```python
from build123d import *

# Parameters (mm, degrees)
F0_W     = 3.0607780209
F0_H     = 2.1009956449
F1_DEPTH = 5
F3_DEPTH = 2
F4_START = -3
F4_DEPTH = 2


with BuildPart() as f1:
    # F0 (on Front) → F1 (new body)
    with BuildSketch(Plane.XZ):
        with BuildLine():
            Line((-13.4510826319, 3.0807058793), (-20.9973859143, 3.0807058793))
            Line((-20.9973859143, 3.0807058793), (-26.770388545, -8.5309240967))
            Line((-26.770388545, -8.5309240967), (-26.3940021396, -8.5309240967))
            Line((-26.3940021396, -8.5309240967), (-26.3940021396, -9.6365026161))
            Line((-26.3940021396, -9.6365026161), (-21.3870331645, -9.6365026161))
            Line((-21.3870331645, -9.6365026161), (-21.3870331645, -11.8402632847))
            Line((-21.3870331645, -11.8402632847), (-24.6597826481, -11.8402632847))
            Line((-24.6597826481, -11.8402632847), (-24.6597826481, -10.3107876107))
            Line((-24.6597826481, -10.3107876107), (-26.3940021396, -10.3107876107))
            Line((-26.3940021396, -10.3107876107), (-26.3940021396, -12.9192377403))
            Line((-26.3940021396, -12.9192377403), (-20.359800871, -12.9192377403))
            ThreePointArc((-20.359800871, -12.9192377403), (-19.8294707851, -12.6995678262), (-19.609800871, -12.1692377403))
            Line((-19.609800871, -12.1692377403), (-19.609800871, -9.2809240967))
            ThreePointArc((-19.609800871, -9.2809240967), (-19.8294707851, -8.7505940108), (-20.359800871, -8.5309240967))
            Line((-20.359800871, -8.5309240967), (-19.2351932671, -8.5309240967))
            Line((-19.2351932671, -8.5309240967), (-16.9493351132, -3.8456239272))
            Line((-16.9493351132, -3.8456239272), (-13.144302211, -8.5309240967))
            Line((-13.144302211, -8.5309240967), (-14.130868949, -8.5309240967))
            Line((-14.130868949, -8.5309240967), (-14.130868949, -11.8141257167))
            Line((-14.130868949, -11.8141257167), (-17.3050090671, -11.8141257167))
            Line((-17.3050090671, -11.8141257167), (-17.3050090671, -8.5309240967))
            Line((-17.3050090671, -8.5309240967), (-19.167387858, -8.5309240967))
            Line((-19.167387858, -8.5309240967), (-19.167387858, -12.1691745073))
            ThreePointArc((-19.167387858, -12.1691745073), (-18.9477179439, -12.6995045932), (-18.417387858, -12.9191745073))
            Line((-18.417387858, -12.9191745073), (-12.2846849263, -12.9191745073))
            Line((-12.2846849263, -12.9191745073), (-12.2846849263, -8.5309240967))
            Line((-12.2846849263, -8.5309240967), (-11.065042235, -8.5309240967))
            ThreePointArc((-11.065042235, -8.5309240967), (-11.5953723208, -8.7505940108), (-11.815042235, -9.2809240967))
            Line((-11.815042235, -9.2809240967), (-11.815042235, -12.1692377403))
            ThreePointArc((-11.815042235, -12.1692377403), (-11.5953723208, -12.6995678262), (-11.065042235, -12.9192377403))
            Line((-11.065042235, -12.9192377403), (-5.1752589643, -12.9192377403))
            Line((-5.1752589643, -12.9192377403), (-5.1752589643, -11.9112924635))
            Line((-5.1752589643, -11.9112924635), (-10.0498311222, -11.9112924635))
            Line((-10.0498311222, -11.9112924635), (-10.0498311222, -9.8059958741))
            Line((-10.0498311222, -9.8059958741), (-5.1752589643, -9.8059958741))
            Line((-5.1752589643, -9.8059958741), (-5.1752589643, -8.5309240967))
            Line((-5.1752589643, -8.5309240967), (-4.6894219704, -8.5309240967))
            Line((-4.6894219704, -8.5309240967), (-4.6894219704, -12.9192377403))
            Line((-4.6894219704, -12.9192377403), (-2.891822136, -12.9192377403))
            Line((-2.891822136, -12.9192377403), (-2.891822136, -11.6197903603))
            Line((-2.891822136, -11.6197903603), (0.1689558849, -11.6197903603))
            Line((0.1689558849, -11.6197903603), (0.1689558849, -12.9192377403))
            Line((0.1689558849, -12.9192377403), (2.096112119, -12.9192377403))
            Line((2.096112119, -12.9192377403), (2.096112119, -8.5309240967))
            Line((2.096112119, -8.5309240967), (2.4571896065, -8.5309240967))
            Line((2.4571896065, -8.5309240967), (7.3034735397, -4.2975358665))
            Line((7.3034735397, -4.2975358665), (6.7291194573, -8.5309240967))
            Line((6.7291194573, -8.5309240967), (3.2661118247, -8.5309240967))
            ThreePointArc((3.2661118247, -8.5309240967), (2.7357817388, -8.7505940108), (2.5161118247, -9.2809240967))
            Line((2.5161118247, -9.2809240967), (2.5161118247, -12.1692377403))
            ThreePointArc((2.5161118247, -12.1692377403), (2.7357817388, -12.6995678262), (3.2661118247, -12.9192377403))
            Line((3.2661118247, -12.9192377403), (9.1558950953, -12.9192377403))
            Line((9.1558950953, -12.9192377403), (9.1558950953, -11.9984643534))
            Line((9.1558950953, -11.9984643534), (4.2813229375, -11.9984643534))
            Line((4.2813229375, -11.9984643534), (4.2813229375, -11.445844546))
            Line((4.2813229375, -11.445844546), (8.6850486696, -11.445844546))
            Line((8.6850486696, -11.445844546), (8.6850486696, -10.4135535657))
            Line((8.6850486696, -10.4135535657), (4.2813229375, -10.4135535657))
            Line((4.2813229375, -10.4135535657), (4.2813229375, -9.805932641))
            Line((4.2813229375, -9.805932641), (9.1558950953, -9.805932641))
            Line((9.1558950953, -9.805932641), (9.1558950953, -8.5309240967))
            Line((9.1558950953, -8.5309240967), (10.1831596047, -8.5309240967))
            ThreePointArc((10.1831596047, -8.5309240967), (9.6528295188, -8.7505940108), (9.4331596047, -9.2809240967))
            Line((9.4331596047, -9.2809240967), (9.4331596047, -10.550885953))
            ThreePointArc((9.4331596047, -10.550885953), (9.6528295188, -11.0812160389), (10.1831596047, -11.300885953))
            Line((10.1831596047, -11.300885953), (14.1622014344, -11.300885953))
            Line((14.1622014344, -11.300885953), (14.1622014344, -11.9984643534))
            Line((14.1622014344, -11.9984643534), (9.4331596047, -11.9984643534))
            Line((9.4331596047, -11.9984643534), (9.4331596047, -12.9191745073))
            Line((9.4331596047, -12.9191745073), (15.0284558833, -12.9191745073))
            ThreePointArc((15.0284558833, -12.9191745073), (15.5587859692, -12.6995045932), (15.7784558833, -12.1691745073))
            Line((15.7784558833, -12.1691745073), (15.7784558833, -11.1678693146))
            ThreePointArc((15.7784558833, -11.1678693146), (15.5587859692, -10.6375392287), (15.0284558833, -10.4178693146))
            Line((15.0284558833, -10.4178693146), (11.2140327692, -10.4178693146))
            Line((11.2140327692, -10.4178693146), (11.2140327692, -9.7743598744))
            Line((11.2140327692, -9.7743598744), (15.7784558833, -9.7743598744))
            Line((15.7784558833, -9.7743598744), (15.7784558833, -8.5309240967))
            Line((15.7784558833, -8.5309240967), (12.7156563103, -8.5309240967))
            Line((12.7156563103, -8.5309240967), (17.5534840673, -4.2975358665))
            Line((17.5534840673, -4.2975358665), (17.0895829797, -8.5309240967))
            Line((17.0895829797, -8.5309240967), (17.0398395211, -8.5309240967))
            ThreePointArc((17.0398395211, -8.5309240967), (16.5095094352, -8.7505940108), (16.2898395211, -9.2809240967))
            Line((16.2898395211, -9.2809240967), (16.2898395211, -10.550885953))
            ThreePointArc((16.2898395211, -10.550885953), (16.5095094352, -11.0812160389), (17.0398395211, -11.300885953))
            Line((17.0398395211, -11.300885953), (21.0188813508, -11.300885953))
            Line((21.0188813508, -11.300885953), (21.0188813508, -11.9984643534))
            Line((21.0188813508, -11.9984643534), (16.2898395211, -11.9984643534))
            Line((16.2898395211, -11.9984643534), (16.2898395211, -12.9191745073))
            Line((16.2898395211, -12.9191745073), (21.8851357996, -12.9191745073))
            ThreePointArc((21.8851357996, -12.9191745073), (22.4154658855, -12.6995045932), (22.6351357996, -12.1691745073))
            Line((22.6351357996, -12.1691745073), (22.6351357996, -11.1678693146))
            ThreePointArc((22.6351357996, -11.1678693146), (22.4154658855, -10.6375392287), (21.8851357996, -10.4178693146))
            Line((21.8851357996, -10.4178693146), (18.0707126856, -10.4178693146))
            Line((18.0707126856, -10.4178693146), (18.0707126856, -9.7743598744))
            Line((18.0707126856, -9.7743598744), (22.6351357996, -9.7743598744))
            Line((22.6351357996, -9.7743598744), (22.6351357996, -8.5309240967))
            Line((22.6351357996, -8.5309240967), (23.4516598284, -8.5309240967))
            Line((23.4516598284, -8.5309240967), (25.7711652666, 3.0807058793))
            Line((25.7711652666, 3.0807058793), (19.431181252, 3.0807058793))
            Line((19.431181252, 3.0807058793), (14.2619935796, -1.4036741341))
            Line((14.2619935796, -1.4036741341), (15.0130717084, 3.0807058793))
            Line((15.0130717084, 3.0807058793), (9.1148968786, 3.0807058793))
            Line((9.1148968786, 3.0807058793), (1.9796516281, -3.5022755619))
            Line((1.9796516281, -3.5022755619), (5.0060558133, 4.4282288291))
            Line((5.0060558133, 4.4282288291), (15.0130717084, 4.4282288291))
            Line((15.0130717084, 4.4282288291), (15.7288057171, 6.8140071817))
            Line((15.7288057171, 6.8140071817), (-11.583940126, 6.8140071817))
            Line((-11.583940126, 6.8140071817), (-12.7105582505, 4.4282288291))
            Line((-12.7105582505, 4.4282288291), (-2.5268180761, 4.4282288291))
            Line((-2.5268180761, 4.4282288291), (-6.9228359498, -5.4683336057))
            Line((-6.9228359498, -5.4683336057), (-10.288979272, -1.3234569953))
            Line((-10.288979272, -1.3234569953), (-4.2719710618, 3.0807058793))
            Line((-4.2719710618, 3.0807058793), (-9.4190677628, 3.0807058793))
            Line((-9.4190677628, 3.0807058793), (-15.5823286623, -1.0281349532))
            Line((-15.5823286623, -1.0281349532), (-13.4510826319, 3.0807058793))
        make_face()
        with Locations((-1.3614331256, -9.5814219192)):
            Rectangle(F0_W, F0_H, mode=Mode.SUBTRACT)
    extrude(amount=F1_DEPTH)

    # F2 (on face) → F3 (cut)
    with BuildSketch(Plane.XZ.offset(5)):
        Polygon((-26.770388545, 6.8140071817), (-26.770388545, -8.5309240967), (26.5221912414, -8.5309240967), (26.5221912414, 6.8140071817), (13.7877286713, 6.8140071817), (7.3034735397, 6.8140071817), (5.1193437539, 6.8140071817), (4.2332103827, 6.8140071817), (2.1055981025, 6.8140071817), (-2.0268179942, 6.8140071817), (-4.4263883249, 6.8140071817), (-10.9106434565, 6.8140071817), align=None)
        Polygon((-5.7986674306, 17.639362709), (-10.9106434565, 6.8140071817), (-4.4263883249, 6.8140071817), (-1.1687912286, 13.7124446064), (-5.4921403697, 13.7124446064), (-4.4917744037, 15.8308655821), (-0.1684252625, 15.8308655821), (0.685587701, 17.639362709), align=None)
        Polygon((-7.9570718311, 8.492592384), (-6.3421407991, 11.9124446064), (-3.5912522867, 11.9124446064), (-5.2061833186, 8.492592384), align=None, mode=Mode.SUBTRACT)
        Polygon((7.3034735397, 6.8140071817), (13.7877286713, 6.8140071817), (18.8997046972, 17.639362709), (12.4154495655, 17.639362709), align=None)
        Polygon((10.0692709763, 8.492592384), (13.3818611683, 15.5074857175), (15.9919188063, 15.5074857175), (12.6793286143, 8.492592384), align=None, mode=Mode.SUBTRACT)
        Polygon((-0.6024195059, 9.8303789273), (-2.0268179942, 6.8140071817), (2.1055981025, 6.8140071817), (4.2332103827, 6.8140071817), (5.1193437539, 6.8140071817), (10.2313197798, 17.639362709), (3.0851580317, 17.639362709), (0.3012099711, 11.7439462647), (5.3197594389, 11.7439462647), (3.7843971086, 8.492592384), (0.9204373378, 8.492592384), (1.5521701913, 9.8303789273), align=None)
        Polygon((2.98915204, 13.6170848409), (3.9799346353, 15.7152116299), (7.1950801421, 15.7152116299), (6.2042975468, 13.6170848409), align=None, mode=Mode.SUBTRACT)
    extrude(amount=-F3_DEPTH, mode=Mode.SUBTRACT)

    # F2 (on face) → F4 (join)
    with BuildSketch(Plane.XZ.offset(5).offset(F4_START)):
        Polygon((-5.7986674306, 17.639362709), (-10.9106434565, 6.8140071817), (-4.4263883249, 6.8140071817), (-1.1687912286, 13.7124446064), (-5.4921403697, 13.7124446064), (-4.4917744037, 15.8308655821), (-0.1684252625, 15.8308655821), (0.685587701, 17.639362709), align=None)
        Polygon((-7.9570718311, 8.492592384), (-6.3421407991, 11.9124446064), (-3.5912522867, 11.9124446064), (-5.2061833186, 8.492592384), align=None, mode=Mode.SUBTRACT)
        Polygon((-0.6024195059, 9.8303789273), (-2.0268179942, 6.8140071817), (2.1055981025, 6.8140071817), (4.2332103827, 6.8140071817), (5.1193437539, 6.8140071817), (10.2313197798, 17.639362709), (3.0851580317, 17.639362709), (0.3012099711, 11.7439462647), (5.3197594389, 11.7439462647), (3.7843971086, 8.492592384), (0.9204373378, 8.492592384), (1.5521701913, 9.8303789273), align=None)
        Polygon((2.98915204, 13.6170848409), (3.9799346353, 15.7152116299), (7.1950801421, 15.7152116299), (6.2042975468, 13.6170848409), align=None, mode=Mode.SUBTRACT)
        Polygon((12.4154495655, 17.639362709), (7.3034735397, 6.8140071817), (13.7877286713, 6.8140071817), (18.8997046972, 17.639362709), align=None)
        Polygon((10.0692709763, 8.492592384), (13.3818611683, 15.5074857175), (15.9919188063, 15.5074857175), (12.6793286143, 8.492592384), align=None, mode=Mode.SUBTRACT)
    extrude(amount=-F4_DEPTH)


solid = f1.part
```
Design review of the part built by this model. Coordinates are the model's own, in mm. A direction names the side the tool comes from. Give positions to 0.01 mm unless a question says otherwise; leave off trailing zeros. Write each loop counter-clockwise with the first axis right and the second up, starting at its lowest first coordinate (ties: lowest second). Pieces come first, ordered by that corner, then holes. Notation, with made-up numbers: (-10, 48.5) - (44, 48.5) arc R19 ccw to (44, 52.5) - close; hole circle Ø9 at (-40, -36.5). An arc over 180 degrees is marked (long way). Return JSON: item names as keys, results as strings. Group by question number.
(1) Insertion check: pin 1 (5 mm diameter, centred on x = 16, z = 3.5, fed in from -Y); pin 2 (0.6 mm diameter, centred on y = -2.5, z = -12.5, fed in from +X); pin 3 (3 mm diameter, centred on y = -3, z = 3.5, fed in from -X). Each pin has a flat end and moves straight along its axis. Give the tip position at first contact, or say it passes through.
(2) To check wall thickness, follow probe 1 along Z at (x, y) = (20, -0.35); probe 2 along Z at (x, y) = (11, -4.4); probe 3 along X at (y, z) = (-0.45, 14.5). State the ranges of each line that lie inside material, in increasing order.
(3) We need section A-A, the plane z = 9. Give the boundary of the cut face in (x, y).
(4) We need section C-C, the plane z = -2. Give the boundary of the cut face in (x, y).
(5) Mouldability with a two-part tool opening along Z and no side actions: class faces 1 (the flat face through (-3, -1, 17.639)), 2 (the flat face through (12, -2, -11.998)), 3 (the flat face through (-9, -5, -9)) as +Z half, -Z half, draft (parallel to the pull), parting line (faces both ways), or undercut.
(6) Machinability: for faces 4 (the flat face through (15.101, -1.479, -6.444)), 5 (the flat face through (4, -2, 12)), 6 (the flat face through (22.635, -2, -12)), 7 (the flat face through (9.156, -2, -9)), which of the approach directions +Z, -Z, +X, -X, +Y, -Y give a long, thin tool a straight path to every point of the face, cutting with its end or side? Answer none if there is none.
(7) We need section B-B, the plane y = -3.5. Give the number of separate pieces and of enclosed holes in the cut face, then the cut area to 3 significant figures.
Reported:
{
 "1": {"pin 1": "stops at y = -3", "pin 2": "stops at x = 22.63", "pin 3": "stops at x = -21.53"},
 "2": {"probe 1": "z = -12.92 to -12, -11.3 to -10.42, -9.77 to 3.08", "probe 2": "z = -12.92 to -12, -11.3 to -8.53", "probe 3": "x = -7.28 to -5.12, 1.6 to 3.41, 6.62 to 8.75, 10.93 to 12.91, 15.52 to 17.42"},
 "3": {"outline": "(-9.88, -2) - (-7.72, -2) - (-7.72, 0) - (-9.88, 0) - close; (-4.97, -2) - (-3.39, -2) - (-3.39, 0) - (-4.97, 0) - close; (-0.99, -2) - (1.16, -2) - (1.16, 0) - (-0.99, 0) - close; (4.02, -2) - (6.15, -2) - (6.15, 0) - (4.02, 0) - close; (8.34, -2) - (10.31, -2) - (10.31, 0) - (8.34, 0) - close; (12.92, -2) - (14.82, -2) - (14.82, 0) - (12.92, 0) - close"},
 "4": {"outline": "(-23.52, -3) - (-9.74, -3) - (-9.74, 0) - (-23.52, 0) - close; (-5.38, -3) - (2.55, -3) - (2.55, 0) - (-5.38, 0) - close; (3.61, -3) - (24.76, -3) - (24.76, 0) - (3.61, 0) - close"},
 "5": {"face 1": "+Z half", "face 2": "undercut", "face 3": "draft"},
 "6": {"face 4": "+Y, -Y", "face 5": "+Z, +X, -X, -Y", "face 6": "-Z, +X, +Y, -Y", "face 7": "-Z, +Y, -Y"},
 "7": {"separate pieces": "7", "enclosed holes": "0", "area": "144 mm2"}
}
